Geometry check sheet. Reference: the model listing, model coordinates, mm. A direction names the side the tool comes from. Round coordinates to 2 decimals unless told otherwise and drop trailing zeros. Write each loop counter-clockwise with the first axis right and the second up, starting at its lowest first coordinate (ties: lowest second). Pieces come first, ordered by that corner, then holes. Notation, with made-up numbers: (2.5, 56) - (8.5, 56) arc R11 cw to (8.5, 72) - close; hole circle Ø10 at (-9, 87.5). An arc over 180 degrees is marked (long way). One line per question, with ' | ' between items. Start each with the question number.
from build123d import *

# Parameters (mm, degrees)
F1_DEPTH    = 2.5
F2_R        = 5
F3_T1_DEPTH = 6.2430809658
F3_T3_DEPTH = 8.6803398875
F3_T5_DEPTH = 12.5


# Not quite as in the source:
# - a fillet or chamfer that OpenCascade refuses, or shapes differently, is made with other operations: its cross-section is extruded or revolved along the edge and cut away or added


with BuildPart() as f1:
    # F0 (on Front) → F1 (new body)
    with BuildSketch(Plane.XZ):
        with BuildLine():
            ThreePointArc((-2, 0), (0.5, 1.9364916731), (1.75, -0.9682458366))
            Line((1.75, -0.9682458366), (1, -3.8729833462))
            Line((1, -3.8729833462), (2, -5.8729833462))
            Line((2, -5.8729833462), (4, -5.8729833462))
            Line((4, -5.8729833462), (4, 0))
            ThreePointArc((4, 0), (0, 4), (-4, 0))
            Line((-4, 0), (-4, -10))
            Line((-4, -10), (2, -17.2908526251))
            Line((2, -17.2908526251), (2, -30))
            ThreePointArc((2, -30), (-0.0346553957, -31.9996997283), (-1.9987990036, -29.9306996147))
            Line((-1.9987990036, -29.9306996147), (-1.9987990036, -17.7522518683))
            Line((-1.9987990036, -17.7522518683), (-4, -14))
            Line((-4, -14), (-4, -30))
            ThreePointArc((-4, -30), (0, -34), (4, -30))
            Line((4, -30), (4, -15))
            Line((4, -15), (-2, -7.7091473749))
            Line((-2, -7.7091473749), (-2, 0))
        make_face()
    extrude(amount=F1_DEPTH)

    # F2
    f2_edges = [f1.edges().sort_by_distance(p)[0] for p in [
        (-4, -1.25, -10),
        (2, -1.25, -17.290853),
        (4, -1.25, -15),
        (-2, -1.25, -7.709147),
        (-1.998799, -1.25, -17.752252),
    ]]
    fillet(f2_edges, radius=F2_R)

    # F3: fillet of radius 2 on 3 edges, made by hand

    # F3_s2 → F3_t1 (cut)
    with BuildSketch(Plane.XZ.offset(-1.8715404829)):
        with BuildLine():
            ThreePointArc((1.1871540483, -3.148138834), (1.1347622142, -3.8587151733), (1.3347913394, -4.542566025))
            Line((1.3347913394, -4.542566025), (1, -3.8729833462))
            Line((1, -3.8729833462), (1.1871540483, -3.148138834))
        make_face()
    extrude(amount=F3_T1_DEPTH, mode=Mode.SUBTRACT)

    # F3_s4 → F3_t3 (cut)
    with BuildSketch(Plane.XZ.offset(-3.0901699437)):
        with BuildLine():
            ThreePointArc((1.4472135955, -4.7674105372), (2.1846057533, -5.5742849629), (3.2360679775, -5.8729833462))
            Line((3.2360679775, -5.8729833462), (2, -5.8729833462))
            Line((2, -5.8729833462), (1.4472135955, -4.7674105372))
        make_face()
    extrude(amount=F3_T3_DEPTH, mode=Mode.SUBTRACT)

    # F3_s6 → F3_t5 (cut)
    with BuildSketch(Plane.XZ.offset(-5)):
        with BuildLine():
            ThreePointArc((2, -5.8729833462), (3.4142135624, -5.2871969086), (4, -3.8729833462))
            Line((4, -3.8729833462), (4, -5.8729833462))
            Line((4, -5.8729833462), (2, -5.8729833462))
        make_face()
    extrude(amount=F3_T5_DEPTH, mode=Mode.SUBTRACT)


solid = f1.part
Q1. Section check B-B, the plane x = -1.5. Record the cut outline in (y, z).
Q2. Draft check along X on faces 1 (the cylindrical face through (3.715, -1.268, -15.128)), 2 (the flat face through (-4, -1, -4)), 3 (the cylindrical face through (0, -1, -32)), 4 (the flat face through (-1.999, -1, -25)). Enter one of: pulls with the +X half, pulls with the -X half, needs draft (parallel to the pull), parting line crosses it, or undercut.
Q3. Thickness scan on line 1 (Z direction, x = 0, y = -1.75); line 2 (X direction, y = -2.2, z = -26.5); line 3 (Z direction, x = -1.5, y = -1.1). Record the ranges inside material, lowest first.
Q4. Section check C-C, the plane x = 3.25. Record the cut outline in (y, z), then the cut area to 3 significant figures.
Q5. Set-up check for faces 5 (the flat face through (-4, -1, -22)), 6 (the cylindrical face through (1.92, -1.23, -5.38)), 7 (the cylindrical face through (-1.698, -1.268, -7.627)): record each of +Z, -Z, +X, -X, +Y, -Y from which the full face is reachable in a straight line by a thin tool's end or side.
Q6. Section check D-D, the plane y = -1.5. Record the cut outline in (x, z), then the cut area to 3 significant figures.
Q7. Section check A-A, the plane z = -23.5. Record the cut outline in (x, y), then the cut area to 3 significant figures.
Result sheet:
1) outline: (-2.5, -33.71) - (0, -33.71) - (0, -31.32) - (-2.5, -31.32) - close; (-2.5, -13.04) - (0, -13.04) - (0, -8.1) - (-2.5, -8.1) - close; (-2.5, 1.32) - (0, 1.32) - (0, 3.71) - (-2.5, 3.71) - close
2) face 1: pulls with the +X half | face 2: pulls with the -X half | face 3: undercut | face 4: undercut
3) line 1: -34 to -32, -14.86 to -10.14, 2 to 4 | line 2: -4 to -2, 2 to 4 | line 3: -33.71 to -31.32, -13.04 to -8.1, 1.32 to 3.71
4) outline: (-2.5, -32.33) - (0, -32.33) - (0, -14.16) - (-2.5, -14.16) - close; (-2.5, -5.43) - (0, -5.43) - (0, 2.33) - (-2.5, 2.33) - close | area: 64.8 mm²
5) face 5: +Z, -Z, -X, +Y, -Y | face 6: +Y, -Y | face 7: +X, +Y, -Y
6) outline: (-4, -30) arc R4 ccw to (4, -30) - (4, -16.79) arc R5 ccw to (2.86, -13.62) - (-0.86, -9.09) arc R5 cw to (-2, -5.92) - (-2, 0) arc R2 cw (long way) to (1.75, -0.97) - (1.19, -3.15) arc R2 ccw to (1.33, -4.54) - (1.45, -4.77) arc R2 ccw to (2.62, -5.78) arc R2 ccw to (4, -3.87) - (4, 0) arc R4 ccw to (-4, 0) - (-4, -8.21) arc R5 ccw to (-2.86, -11.38) - (0.86, -15.91) arc R5 cw to (2, -19.08) - (2, -30) arc R2 cw (long way) to (-2, -29.93) - (-2, -19) arc R5 ccw to (-2.59, -16.65) - (-4, -14) - close | area: 153 mm²
7) outline: (-4, -2.5) - (-2, -2.5) - (-2, 0) - (-4, 0) - close; (2, -2.5) - (4, -2.5) - (4, 0) - (2, 0) - close | area: 10.0 mm²
